Work out the finished part from the listing and answer in its coordinate system (mm). A direction names the side the tool comes from. Coordinates: 2 decimals unless noted, no trailing zeros. Order: outer loops, then holes, each group sorted by start corner. A loop starts at its lowest first (then second) coordinate and runs counter-clockwise, first axis right, second up. Notation, with made-up numbers: M 58,33.25 L 73,33.25 A8 ccw 73,46.25 Z; hole C 23.5,48 d10. An arc over 180 degrees is marked long. Use a Markdown table: item, result.
from build123d import *

# Parameters (mm, degrees)
SKETCH_1_W      = 41
SKETCH_1_H      = 90
SKETCH_1_R      = 1.25
SKETCH_1_R_2    = 1.75
EXTRUDE_1_DEPTH = 3
FILLET_1_R      = 2
FILLET_2_R      = 5
FILLET_3_R      = 2


with BuildPart() as part:
    # 草图1 → 凸台-拉伸1 (new body)
    with BuildSketch(Plane(origin=(0, 0, 0), x_dir=(1, 0, 0), z_dir=(0, 1, 0))):
        Polygon((-28.5, -37.5), (-41.5, -37.5), (-41.5, -45), (-28.5, -45), (-28.5, -56), (28.5, -56), (28.5, -45), (41.5, -45), (41.5, -37.5), (28.5, -37.5), (28.5, -14.9), (41.5, -14.9), (41.5, 14.9), (28.5, 14.9), (28.5, 37.5), (41.5, 37.5), (41.5, 45), (28.5, 45), (28.5, 56), (-28.5, 56), (-28.5, 45), (-41.5, 45), (-41.5, 37.5), (-28.5, 37.5), (-28.5, 14.9), (-41.5, 14.9), (-41.5, -14.9), (-28.5, -14.9), align=None)
        Rectangle(SKETCH_1_W, SKETCH_1_H, mode=Mode.SUBTRACT)
        with Locations((-35, -39.95)):
            Circle(SKETCH_1_R, mode=Mode.SUBTRACT)
        with Locations((18.5, -49)):
            Circle(SKETCH_1_R_2, mode=Mode.SUBTRACT)
        with Locations((-18.5, -49)):
            Circle(SKETCH_1_R_2, mode=Mode.SUBTRACT)
        with Locations((-36, 12.45)):
            Circle(SKETCH_1_R, mode=Mode.SUBTRACT)
        with Locations((-36, -12.45)):
            Circle(SKETCH_1_R, mode=Mode.SUBTRACT)
        with Locations((0, -49)):
            Circle(SKETCH_1_R_2, mode=Mode.SUBTRACT)
        with Locations((18.5, 49)):
            Circle(SKETCH_1_R_2, mode=Mode.SUBTRACT)
        with Locations((-18.5, 49)):
            Circle(SKETCH_1_R_2, mode=Mode.SUBTRACT)
        with Locations((0, 49)):
            Circle(SKETCH_1_R_2, mode=Mode.SUBTRACT)
        with Locations((-35, 39.95)):
            Circle(SKETCH_1_R, mode=Mode.SUBTRACT)
        with Locations((35, 39.95)):
            Circle(SKETCH_1_R, mode=Mode.SUBTRACT)
        with Locations((35, -39.95)):
            Circle(SKETCH_1_R, mode=Mode.SUBTRACT)
        with Locations((36, 12.45)):
            Circle(SKETCH_1_R, mode=Mode.SUBTRACT)
        with Locations((36, -12.45)):
            Circle(SKETCH_1_R, mode=Mode.SUBTRACT)
    extrude(amount=EXTRUDE_1_DEPTH)

    # 圆角1
    fillet_1_edges = [part.edges().sort_by_distance(p)[0] for p in [
        (-41.5, 1.5, 45),
        (-41.5, 1.5, 37.5),
        (-41.5, 1.5, 14.9),
        (-41.5, 1.5, -14.9),
        (-41.5, 1.5, -37.5),
        (-41.5, 1.5, -45),
        (41.5, 1.5, -45),
        (41.5, 1.5, -37.5),
        (41.5, 1.5, -14.9),
        (41.5, 1.5, 14.9),
        (41.5, 1.5, 37.5),
        (41.5, 1.5, 45),
    ]]
    fillet(fillet_1_edges, radius=FILLET_1_R)

    # 圆角2
    fillet_2_edges = [part.edges().sort_by_distance(p)[0] for p in [
        (28.5, 1.5, 56),
        (-28.5, 1.5, 56),
        (-28.5, 1.5, -56),
        (28.5, 1.5, -56),
        (20.5, 1.5, 45),
        (20.5, 1.5, -45),
        (-20.5, 1.5, -45),
        (-20.5, 1.5, 45),
    ]]
    fillet(fillet_2_edges, radius=FILLET_2_R)

    # 圆角3
    fillet_3_edges = [part.edges().sort_by_distance(p)[0] for p in [
        (-28.5, 1.5, 45),
        (-28.5, 1.5, -45),
        (28.5, 1.5, -45),
        (28.5, 1.5, 45),
    ]]
    fillet(fillet_3_edges, radius=FILLET_3_R)


solid = part.part
(1) Which of the six approach directions +Z, -Z, +X, -X, +Y, -Y give full straight-line access (tool end or side, diameter ignored) to faces 4 (the flat face through (34, 1, 37.5)), 5 (the flat face through (-34, 1, 37.5)), 6 (the flat face through (35, 1, 45)), 7 (the flat face through (-20.5, 1, 1))?
Conclusion:
| item | result |
|---|---|
| face 4 | +X, +Y, -Y |
| face 5 | -X, +Y, -Y |
| face 6 | +Z, +X, +Y, -Y |
| face 7 | +Y, -Y |
(2) Straight lines are drawn through the part: L1, parallel to X at y = 1.6, z = 49; L2, parallel to X at y = 1.35, z = -39.95; L3, parallel to Z at x = 0, y = 0.85. For each, find the intervals that lie inside material, in ascending order.
Conclusion:
| item | result |
|---|---|
| L1 | -28.5 to -20.25, -16.75 to -1.75, 1.75 to 16.75, 20.25 to 28.5 |
| L2 | -41.5 to -36.25, -33.75 to -20.5, 20.5 to 33.75, 36.25 to 41.5 |
| L3 | -56 to -50.75, -47.25 to -45, 45 to 47.25, 50.75 to 56 |
(3) Determine the mould class of faces 1 (the cylindrical face through (-18.88, 1.48, -47.29)), 2 (the flat face through (-35, 1, 45)), 3 (the flat face through (41.5, 1, -41)) for opening direction Z: pulls with the +Z half, pulls with the -Z half, needs draft (parallel to the pull), parting line crosses it, or undercut.
Conclusion:
| item | result |
|---|---|
| face 1 | undercut |
| face 2 | pulls with the +Z half |
| face 3 | needs draft |
(4) Given P1, Ø3, axis at x = 36, z = 12.45, coming from the +Y side; P2, Ø0.9, axis at x = -32, y = 2, coming from the +Z side; P3, Ø1.5, axis at x = 32, y = 2, coming from the -Z side, each flat-ended and moving along its own axis, determine where each tip first touches the part or whether it passes through.
Conclusion:
| item | result |
|---|---|
| P1 | y = 3 |
| P2 | z = 45 |
| P3 | z = -45 |
(5) A cutting plane is placed at C-C (z = -1). Determine the outline of the cut face in (x, y), then the cut area to 3 significant figures.
Conclusion:
| item | result |
|---|---|
| outline | M -41.5,0 L -20.5,0 L -20.5,3 L -41.5,3 Z; M 20.5,0 L 41.5,0 L 41.5,3 L 20.5,3 Z |
| area | 126 mm2 |
(6) A cutting plane is placed at B-B (x = 0). Determine the outline of the cut face in (y, z).
Conclusion:
| item | result |
|---|---|
| outline | M 0,-56 L 3,-56 L 3,-50.75 L 0,-50.75 Z; M 0,-47.25 L 3,-47.25 L 3,-45 L 0,-45 Z; M 0,45 L 3,45 L 3,47.25 L 0,47.25 Z; M 0,50.75 L 3,50.75 L 3,56 L 0,56 Z |
(7) A cutting plane is placed at A-A (z = -49). Determine the outline of the cut face in (x, y), then the cut area to 4 significant figures.
Conclusion:
| item | result |
|---|---|
| outline | M -28.5,0 L -20.25,0 L -20.25,3 L -28.5,3 Z; M -16.75,0 L -1.75,0 L -1.75,3 L -16.75,3 Z; M 1.75,0 L 16.75,0 L 16.75,3 L 1.75,3 Z; M 20.25,0 L 28.5,0 L 28.5,3 L 20.25,3 Z |
| area | 139.5 mm2 |
(8) A cutting plane is placed at D-D (y = 0.8). Give the number of separate pieces and of enclosed holes in the cut face, then the cut area to 3 significant figures.
Conclusion:
| item | result |
|---|---|
| separate pieces | 1 |
| enclosed holes | 15 |
| area | 3,750 mm2 |
